Geometry: final body of the model. Coordinates: model frame, mm. A direction names the side the tool comes from. Give positions to 0.01 mm unless a question says otherwise; leave off trailing zeros. Write each loop counter-clockwise with the first axis right and the second up, starting at its lowest first coordinate (ties: lowest second). Pieces come first, ordered by that corner, then holes. Notation, with made-up numbers: (80.25, -5.75) - (89.25, -5.75) arc R16 ccw to (89.25, 3.25) - close; hole circle Ø5 at (-19.75, -29.5). An arc over 180 degrees is marked (long way). Return JSON: item names as keys, results as strings.
from build123d import *

# Parameters (mm, degrees)
SKETCH_1_R               = 16
EXTRUDE_1_DEPTH          = 20
SKETCH_2_R               = 40
EXTRUDE_2_DEPTH          = 26
SKETCH_3_W               = 1
SKETCH_3_H               = 2.5
SKETCH_4_R               = 5
CUT_EXTRUDE_1_DEPTH      = 8
PATTERN_CIRCULAR_1_COUNT = 8
CHAMFER_1_SIZE           = 1
SKETCH_5_R               = 22.5
EXTRUDE_3_DEPTH          = 101
SKETCH_6_R               = 20
EXTRUDE_4_DEPTH          = 40
SKETCH_7_R               = 17.5
EXTRUDE_5_DEPTH          = 79
SKETCH_8_R               = 12.5
EXTRUDE_6_DEPTH          = 26
SKETCH_9_R               = 10
EXTRUDE_7_DEPTH          = 26
CHAMFER_2_SIZE           = 1
CHAMFER_3_SIZE           = 1
SKETCH_10_R              = 2.5
CUT_EXTRUDE_2_DEPTH      = 7


with BuildPart() as part:
    # 草图1 → 凸台-拉伸1 (new body)
    with BuildSketch(Plane.XY):
        Circle(SKETCH_1_R)
    extrude(amount=EXTRUDE_1_DEPTH)

    # 草图2 → 凸台-拉伸2 (add)
    with BuildSketch(Plane(origin=(0, 0, 0), x_dir=(-1, 0, 0), z_dir=(0, 0, -1))):
        Circle(SKETCH_2_R)
    extrude(amount=EXTRUDE_2_DEPTH)

    # 草图3 → 切除-旋转1 (revolve, cut)
    with BuildSketch(Plane(origin=(0, 0, 0), x_dir=(1, 0, 0), z_dir=(0, 1, 0))):
        with Locations((15.5, -13.75)):
            Rectangle(SKETCH_3_W, SKETCH_3_H)
    revolve(axis=Axis((0, 0, 0), (0, 0, 1)), mode=Mode.SUBTRACT)

    # 草图4 → 切除-拉伸1 (cut)
    with BuildSketch(Plane.XY):
        with Locations((28, 0)):
            Circle(SKETCH_4_R)
    cut_extrude_1 = extrude(amount=-CUT_EXTRUDE_1_DEPTH, mode=Mode.SUBTRACT)

    # 阵列(圆周)1: 切除-拉伸1 ×8 about axis
    pattern_circular_1_axis = Axis((0, 0, 0), (0, 0, 1))
    for i in range(1, PATTERN_CIRCULAR_1_COUNT):
        add(cut_extrude_1.rotate(pattern_circular_1_axis, i * 360 / PATTERN_CIRCULAR_1_COUNT), mode=Mode.SUBTRACT)

    # 倒角1
    chamfer_1_edges = [part.edges().sort_by_distance(p)[0] for p in [
        (-16, 0, 20),
    ]]
    chamfer(chamfer_1_edges, length=CHAMFER_1_SIZE)

    # 草图5 → 凸台-拉伸3 (add)
    with BuildSketch(Plane(origin=(0, 0, -26), x_dir=(-1, 0, 0), z_dir=(0, 0, -1))):
        Circle(SKETCH_5_R)
    extrude(amount=EXTRUDE_3_DEPTH)

    # 草图6 → 凸台-拉伸4 (add)
    with BuildSketch(Plane(origin=(0, 0, -127), x_dir=(-1, 0, 0), z_dir=(0, 0, -1))):
        Circle(SKETCH_6_R)
    extrude(amount=EXTRUDE_4_DEPTH)

    # 草图7 → 凸台-拉伸5 (add)
    with BuildSketch(Plane(origin=(0, 0, -167), x_dir=(-1, 0, 0), z_dir=(0, 0, -1))):
        Circle(SKETCH_7_R)
    extrude(amount=EXTRUDE_5_DEPTH)

    # 草图8 → 凸台-拉伸6 (add)
    with BuildSketch(Plane(origin=(0, 0, -246), x_dir=(-1, 0, 0), z_dir=(0, 0, -1))):
        Circle(SKETCH_8_R)
    extrude(amount=EXTRUDE_6_DEPTH)

    # 草图9 → 凸台-拉伸7 (add)
    with BuildSketch(Plane(origin=(0, 0, -272), x_dir=(-1, 0, 0), z_dir=(0, 0, -1))):
        Circle(SKETCH_9_R)
    extrude(amount=EXTRUDE_7_DEPTH)

    # 倒角2
    chamfer_2_edges = [part.edges().sort_by_distance(p)[0] for p in [
        (20, 0, -167),
        (17.5, 0, -246),
        (12.5, 0, -272),
        (10, 0, -298),
    ]]
    chamfer(chamfer_2_edges, length=CHAMFER_2_SIZE)

    # 倒角3
    chamfer_3_edges = [part.edges().sort_by_distance(p)[0] for p in [
        (22.5, 0, -127),
    ]]
    chamfer(chamfer_3_edges, length=CHAMFER_3_SIZE)

    # 草图10 → 切除-拉伸2 (cut)
    with BuildSketch(Plane(origin=(0, 0, -298), x_dir=(-1, 0, 0), z_dir=(0, 0, -1))):
        with Locations((-6, 0.24134819)):
            Circle(SKETCH_10_R)
        with Locations((6, 0)):
            Circle(SKETCH_10_R)
    extrude(amount=-CUT_EXTRUDE_2_DEPTH, mode=Mode.SUBTRACT)


solid = part.part
Q1. Section query D-D, the plane z = -220. Return the cut outline in (x, y).
Answer key:
{"outline": "circle Ø35 at (0, 0)"}
Q2. Material intervals for probe 1 along Z at (x, y) = (-35, -6); probe 2 along Y at (x, z) = (-1, -146); probe 3 along Z at (x, y) = (-23, 22.5), sorted ascending. Write a range as [from, to].
Answer key:
{"probe 1": "z = [-26, 0]", "probe 2": "y = [-19.97, 19.97]", "probe 3": "z = [-26, -8]"}
Q3. Set-up query: faces 4 (the flat face through (-28, 0, -8)), 5 (the cylindrical face through (-10.382, -19.961, -75.3)). Return all of +Z, -Z, +X, -X, +Y, -Y with unobstructed straight access to the full face (end or side cutting, diameter ignored); none if empty.
Answer key:
{"face 4": "+Z", "face 5": "-Z"}
Q4. Pin query (flat end, axial travel): P1, Ø1.5, axis at x = -7, y = -0.5, coming from the -Z side; P2, Ø11, axis at x = -28.5, y = -2, coming from the +Z side; P3, Ø1.5, axis at x = 1, z = -203.5, coming from the +Y side; P4, Ø18.5, axis at x = 4.5, y = 2, coming from the -Z side. Return the tip coordinate at first contact, or that it passes through.
Answer key:
{"P1": "stops at z = -291", "P2": "stops at z = 0", "P3": "stops at y = 17.5", "P4": "stops at z = -298"}
Q5. Section query C-C, the plane z = -115.5. Return the cut outline in (x, y).
Answer key:
{"outline": "circle Ø45 at (0, 0)"}
Q6. Section query A-A, the plane y = -28. Return the cut outline in (x, z).
Answer key:
{"outline": "(-28.57, -26) - (28.57, -26) - (28.57, 0) - (5, 0) - (5, -8) - (-5, -8) - (-5, 0) - (-28.57, 0) - close"}
Q7. Mould query, pull axis X, two halves, no side actions, for faces 1 (the flat face through (0, 0, -298)), 2 (the cylindrical face through (13.887, -10.648, -205.454)), 3 (the flat face through (0, -28, -8)). Classes: pulls with the +X half, pulls with the -X half, needs draft (parallel to the pull), parting line crosses it, or undercut.
Answer key:
{"face 1": "needs draft", "face 2": "parting line crosses it", "face 3": "undercut"}
